The listing builds one solid part. Answer for the finished solid, in the listing's coordinates (mm). A direction names the side the tool comes from. Round coordinates to 2 decimals unless told otherwise and drop trailing zeros. Write each loop counter-clockwise with the first axis right and the second up, starting at its lowest first coordinate (ties: lowest second). Pieces come first, ordered by that corner, then holes.
(1) This flat-tipped pin is pushed along its axis until it touches: pin 1 Ø2.5 at (x, z) = (-108.3, -261.46) entering from -Y. Where does it stop, or does it pass through?
(2) For faces 1 (the face through (-76.43, 1.48, -281.3)), 2 (the face through (-166.91, 1.48, -220.44)), determine the directions among +Z, -Z, +X, -X, +Y, -Y from which every point of the face is accessible in a straight line to the end or side of a thin tool.
(3) The mould has two halves that part along X. Classify faces 3 (the face through (74.46, 1.48, -281.83)), 4 (the face through (1, 0, -274)), 5 (the face through (72.38, 1.48, -266.86)): +X half, -X half, draft (parallel to the pull), parting line (faces both ways), or undercut.
(4) Find the intervals of material crossed by probe 1 along X at (y, z) = (1.5, -247.5); probe 2 along X at (y, z) = (0.4, -248); probe 3 along X at (y, z) = (1.2, -217), in increasing order.
(5) A cutting plane is placed at B-B, the plane x = -133.5. Give the vertices of the cut face in (y, z), and give its area (3 significant figures).
(6) A cutting plane is placed at C-C, the plane y = 1.1. Give the number of separate pieces and of enclosed holes in the cut face, and give its area (3 significant figures).
(7) A cutting plane is placed at A-A, the plane z = -268. Give the vertices of the cut face in (x, y), and give its area (3 significant figures).
(8) A cutting plane is placed at D-D, the plane x = 21. Give the vertices of the cut face in (y, z).
from build123d import *

# Parameters (mm, degrees)
BOSS_EXTRUDE1_DEPTH = 3
FILLET1_R           = 2
FILLET2_R           = 2
FILLET3_R           = 2
BOSS_EXTRUDE2_START = -3
BOSS_EXTRUDE2_DEPTH = 3
FILLET4_R           = 2
SKETCH3_R           = 1.65
CUT_EXTRUDE1_DEPTH  = 10


with BuildPart() as part:
    # Sketch1 → Boss-Extrude1 (new body)
    with BuildSketch(Plane(origin=(0, 0, 0), x_dir=(1, 0, 0), z_dir=(0, 1, 0))):
        with BuildLine():
            Line((-147.176606992, 251.617360996), (-143.528941916, 245.299419756))
            Line((-143.528941916, 245.299419756), (-140.671058084, 246.949419756))
            Line((-140.671058084, 246.949419756), (-144.318723159, 253.267360996))
            ThreePointArc((-144.318723159, 253.267360996), (-75.445751647, 281.567378363), (-1.65, 291.495330151))
            Line((-1.65, 291.495330151), (-1.65, 284.2))
            Line((-1.65, 284.2), (1.65, 284.2))
            Line((1.65, 284.2), (1.65, 291.495330151))
            ThreePointArc((1.65, 291.495330151), (75.445751647, 281.567378363), (144.318723159, 253.267360996))
            Line((144.318723159, 253.267360996), (140.671058084, 246.949419756))
            Line((140.671058084, 246.949419756), (143.528941916, 245.299419756))
            Line((143.528941916, 245.299419756), (147.176606992, 251.617360996))
            ThreePointArc((147.176606992, 251.617360996), (150.840163403, 249.438359329), (154.471465524, 247.20602003))
            Line((154.471465524, 247.20602003), (143.873080239, 230.245058106))
            ThreePointArc((143.873080239, 230.245058106), (135.75, 235.125897127), (127.461529296, 239.720271461))
            Line((127.461529296, 239.720271461), (129.80888711, 244.135009425))
            ThreePointArc((129.80888711, 244.135009425), (71.563465971, 267.078490969), (9.649710838, 276.331563671))
            Line((9.649710838, 276.331563671), (9.475213355, 271.334609536))
            ThreePointArc((9.475213355, 271.334609536), (0, 271.5), (-9.475213355, 271.334609536))
            Line((-9.475213355, 271.334609536), (-9.649710838, 276.331563671))
            ThreePointArc((-9.649710838, 276.331563671), (-71.563465971, 267.078490969), (-129.80888711, 244.135009425))
            Line((-129.80888711, 244.135009425), (-127.461529296, 239.720271461))
            ThreePointArc((-127.461529296, 239.720271461), (-135.75, 235.125897127), (-143.873080239, 230.245058106))
            Line((-143.873080239, 230.245058106), (-154.471465524, 247.20602003))
            ThreePointArc((-154.471465524, 247.20602003), (-150.840163403, 249.438359329), (-147.176606992, 251.617360996))
        make_face()
    extrude(amount=BOSS_EXTRUDE1_DEPTH)

    # Fillet1
    fillet1_edges = [part.edges().sort_by_distance(p)[0] for p in [
        (127.461529296, 1.5, -239.720271461),
        (129.80888711, 1.5, -244.135009425),
        (9.649710838, 1.5, -276.331563671),
        (9.475213355, 1.5, -271.334609536),
        (-9.475213355, 1.5, -271.334609536),
        (-9.649710838, 1.5, -276.331563671),
        (-129.80888711, 1.5, -244.135009425),
        (-127.461529296, 1.5, -239.720271461),
    ]]
    fillet(fillet1_edges, radius=FILLET1_R)

    # Fillet2
    fillet2_edges = [part.edges().sort_by_distance(p)[0] for p in [
        (154.471465524, 1.5, -247.20602003),
        (143.873080239, 1.5, -230.245058106),
        (-143.873080239, 1.5, -230.245058106),
        (-154.471465524, 1.5, -247.20602003),
    ]]
    fillet(fillet2_edges, radius=FILLET2_R)

    # Fillet3
    fillet3_edges = [part.edges().sort_by_distance(p)[0] for p in [
        (-147.176606992, 1.5, -251.617360996),
        (-144.318723159, 1.5, -253.267360996),
        (-1.65, 1.5, -291.495330151),
        (1.65, 1.5, -291.495330151),
        (144.318723159, 1.5, -253.267360996),
        (147.176606992, 1.5, -251.617360996),
    ]]
    fillet(fillet3_edges, radius=FILLET3_R)

    # Sketch2 → Boss-Extrude2 (add)
    with BuildSketch(Plane(origin=(0, 3, 0), x_dir=(1, 0, 0), z_dir=(0, 1, 0)).offset(BOSS_EXTRUDE2_START)):
        with BuildLine():
            Line((-152.759965651, 248.267281159), (-146.52267656, 234.485298587))
            ThreePointArc((-146.52267656, 234.485298587), (-166.367665138, 220.84847746), (-184.950980973, 205.536820636))
            ThreePointArc((-184.950980973, 205.536820636), (-188.514353616, 204.258373219), (-191.95225185, 205.843588702))
            Line((-191.95225185, 205.843588702), (-195.362772292, 209.500924109))
            ThreePointArc((-195.362772292, 209.500924109), (-196.701244935, 213.129011848), (-195.0516583, 216.6266387))
            ThreePointArc((-195.0516583, 216.6266387), (-174.623921622, 233.406803666), (-152.759965651, 248.267281159))
        make_face()
        with BuildLine():
            Line((191.95225185, 205.843588702), (195.362772292, 209.500924109))
            ThreePointArc((195.362772292, 209.500924109), (196.701244935, 213.129011848), (195.0516583, 216.6266387))
            ThreePointArc((195.0516583, 216.6266387), (174.623921622, 233.406803666), (152.759965651, 248.267281159))
            Line((152.759965651, 248.267281159), (146.52267656, 234.485298587))
            ThreePointArc((146.52267656, 234.485298587), (166.367665138, 220.84847746), (184.950980973, 205.536820636))
            ThreePointArc((184.950980973, 205.536820636), (188.514353616, 204.258373219), (191.95225185, 205.843588702))
        make_face()
    extrude(amount=BOSS_EXTRUDE2_DEPTH)

    # Fillet4
    fillet4_edges = [part.edges().sort_by_distance(p)[0] for p in [
        (-146.52267656, 1.5, -234.485298587),
        (146.52267656, 1.5, -234.485298587),
    ]]
    fillet(fillet4_edges, radius=FILLET4_R)

    # Sketch3 → Cut-Extrude1 (cut)
    with BuildSketch(Plane(origin=(0, 3, 0), x_dir=(1, 0, 0), z_dir=(0, 1, 0))):
        with Locations(Location((-36.938912398, 280.578895769, 0), (0, 0, 270))):
            Circle(SKETCH3_R)
        with Locations(Location((36.938912398, 280.578895769, 0), (0, 0, 270))):
            Circle(SKETCH3_R)
        with Locations(Location((108.299411359, 261.457907701, 0), (0, 0, 270))):
            Circle(SKETCH3_R)
        with Locations(Location((-108.299411359, 261.457907701, 0), (0, 0, 270))):
            Circle(SKETCH3_R)
        with Locations(Location((172.279484409, 224.518995302, 0), (0, 0, 270))):
            Circle(SKETCH3_R)
        with Locations(Location((-172.279484409, 224.518995302, 0), (0, 0, 270))):
            Circle(SKETCH3_R)
    extrude(amount=-CUT_EXTRUDE1_DEPTH, mode=Mode.SUBTRACT)


solid = part.part
Solutions:
1. pin 1: passes through
2. face 1: -Z, -X, +Y, -Y
2. face 2: +Z, +Y, -Y
3. face 3: +X half
3. face 4: draft
3. face 5: undercut
4. probe 1: x = -154 to -144.8, -140.99 to -123.27, 123.27 to 140.99, 144.8 to 154
4. probe 2: x = -153.19 to -145.09, -141.28 to -122.26, 122.26 to 141.28, 145.09 to 153.19
4. probe 3: x = -194.64 to -171.36, 171.36 to 194.64
5. outline: (0, -259.13) - (3, -259.13) - (3, -236.41) - (0, -236.41) - close
5. area: 68.2 mm2
6. separate pieces: 1
6. enclosed holes: 6
6. area: 6,530 mm2
7. outline: (-114.67, 0) - (-68.03, 0) - (-68.03, 3) - (-114.67, 3) - close; (68.03, 0) - (114.67, 0) - (114.67, 3) - (68.03, 3) - close
7. area: 280 mm2
8. outline: (0, -290.74) - (3, -290.74) - (3, -275.7) - (0, -275.7) - close
